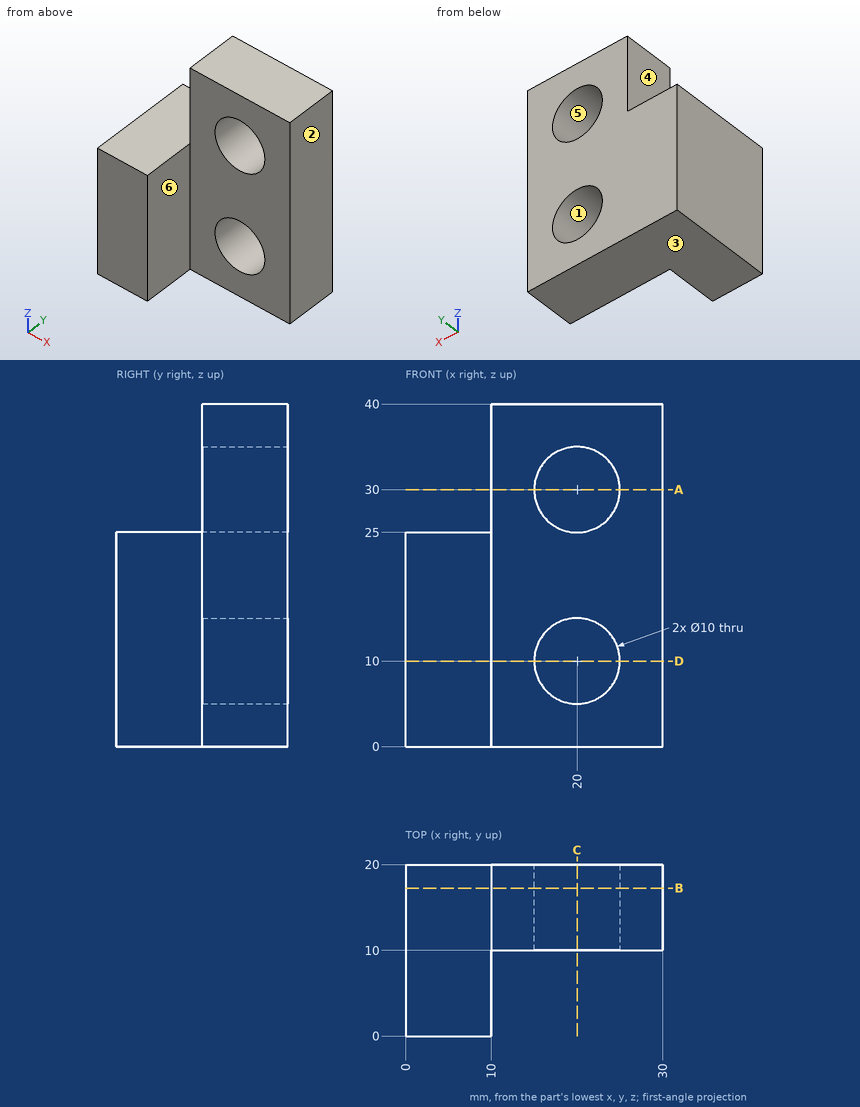
Geometry: see drawing. Coordinates: mm, zero at the bounding-box minimum. A direction names the side the tool comes from. Give positions to 0.01 mm unless a question says otherwise; leave off trailing zeros. Loops run counter-clockwise (first coordinate to the right, second up) from the corner with the lowest first, then second, coordinate; pieces in that order, holes last. Notation, with made-up numbers: (-17.75, 77.25) -> (-6.75, 77.25) arc R16 cw to (-6.75, 91.25) -> close; hole circle Ø10 at (43.5, 77.25). An arc over 180 degrees is marked (long way). Put each result on its own line as item: value.
1. Pull-direction query (X, two-part tool) for the marked faces 1, 2 and 3; classes: released by +X, released by -X, zero draft, split by the parting line, or undercut.
Taken from the geometry:
face 1: undercut
face 2: released by +X
face 3: zero draft
2. Set-up query: the marked faces 4, 5 and 6. Return all of +Z, -Z, +X, -X, +Y, -Y with unobstructed straight access to the full face (end or side cutting, diameter ignored); none if empty.
Taken from the geometry:
face 4: +Z, -X, +Y, -Y
face 5: +Y, -Y
face 6: +Z, -Z, +X, -Y
3. Cut plane C-C (x = 20). Return the cut outline in (y, z), plus the area to 3 significant figures.
Taken from the geometry:
outline: (10, 0) -> (20, 0) -> (20, 5) -> (10, 5) -> close; (10, 15) -> (20, 15) -> (20, 25) -> (10, 25) -> close; (10, 35) -> (20, 35) -> (20, 40) -> (10, 40) -> close
area: 200 mm2
4. Pin query (flat end, axial travel): P1, Ø4, axis at x = 25.5, z = 4.5, coming from the -Y side; P2, Ø12, axis at x = 8.5, z = 21.5, coming from the -Y side; P3, Ø8, axis at x = 20, z = 10, coming from the +Y side; P4, Ø8, axis at y = 3, z = 11, coming from the +X side. Return the tip coordinate at first contact, or that it passes through.
Taken from the geometry:
P1: stops at y = 10
P2: stops at y = 0
P3: passes through
P4: stops at x = 10
5. Cut plane A-A (z = 30). Return the cut outline in (x, y).
Taken from the geometry:
outline: (10, 10) -> (15, 10) -> (15, 20) -> (10, 20) -> close; (25, 10) -> (30, 10) -> (30, 20) -> (25, 20) -> close
6. Ray query, line 1 along Z through (x, y) = (20, 14); line 2 along Z through (x, y) = (6.5, 11.5); line 3 along Z through (x, y) = (21, 15.5). Return the intervals inside material, ascending. Write a range as [from, to].
Taken from the geometry:
line 1: z = [0, 5], [15, 25], [35, 40]
line 2: z = [0, 25]
line 3: z = [0, 5.1], [14.9, 25.1], [34.9, 40]
7. Cut plane D-D (z = 10). Return the cut outline in (x, y), plus the area to 3 significant figures.
Taken from the geometry:
outline: (0, 0) -> (10, 0) -> (10, 10) -> (15, 10) -> (15, 20) -> (0, 20) -> close; (25, 10) -> (30, 10) -> (30, 20) -> (25, 20) -> close
area: 300 mm2
8. Cut plane B-B (y = 17.25). Return the cut outline in (x, z).
Taken from the geometry:
outline: (0, 0) -> (30, 0) -> (30, 40) -> (10, 40) -> (10, 25) -> (0, 25) -> close; hole circle Ø10 at (20, 10); hole circle Ø10 at (20, 30)
